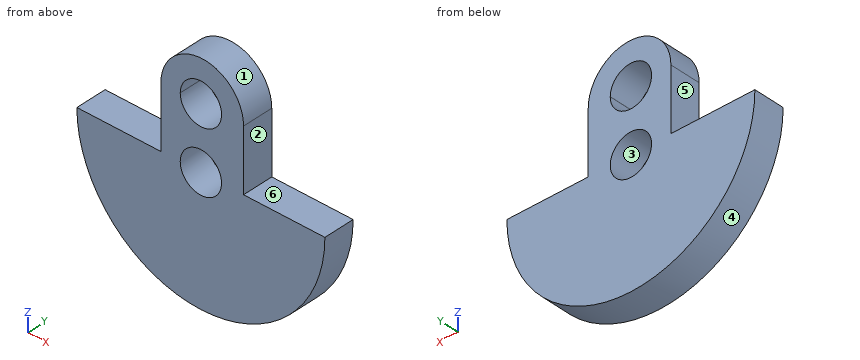
```python
from build123d import *

# Parameters (mm, degrees)
F1_DEPTH = 15


with BuildPart() as f1:
    # F0 (on Front) → F1 (new body)
    with BuildSketch(Plane.XZ):
        with BuildLine():
            Line((-19.364525, 0), (-60, 0))
            ThreePointArc((-60, 0), (0, -60), (60, 0))
            Line((60, 0), (20.64457, 0))
            Line((20.64457, 0), (10, 0))
            ThreePointArc((10, 0), (0, -10), (-10, 0))
            Line((-10, 0), (-19.364525, 0))
        make_face()
        with BuildLine():
            Line((-19.364525, 30.053675), (-19.364525, 0))
            Line((-19.364525, 0), (-10, 0))
            ThreePointArc((-10, 0), (0, 10), (10, 0))
            Line((10, 0), (20.64457, 0))
            Line((20.64457, 0), (20.64457, 30.053675))
            Line((20.64457, 30.053675), (9.999856, 30.053675))
            ThreePointArc((9.999856, 30.053675), (9.999964, 30.026838), (10, 30))
            ThreePointArc((10, 30), (-0.026838, 20.000036), (-9.999856, 30.053675))
            Line((-9.999856, 30.053675), (-19.364525, 30.053675))
        make_face()
        with BuildLine():
            ThreePointArc((20.64457, 30.053675), (0.640023, 50.058223), (-19.364525, 30.053675))
            Line((-19.364525, 30.053675), (-9.999856, 30.053675))
            ThreePointArc((-9.999856, 30.053675), (0, 40), (9.999856, 30.053675))
            Line((9.999856, 30.053675), (20.64457, 30.053675))
        make_face()
    extrude(amount=F1_DEPTH)


solid = f1.part
```
Build history of the part. All positions in model axes, mm. Face numbers are marked on the shaded views. A direction names the side the tool comes from. Round coordinates to 2 decimals unless told otherwise and drop trailing zeros. Write each loop counter-clockwise with the first axis right and the second up, starting at its lowest first coordinate (ties: lowest second). Pieces come first, ordered by that corner, then holes.
1) Band-saw the part on D-D, the plane z = 37.5. List the corners of the cut face in (x, y).
2) Band-saw the part on A-A, the plane y = -4. List the corners of the cut face in (x, z), and give its area (3 significant figures).
3) Pin check, flat tips, straight feed: pin 1 (1 mm diameter, centred on x = 6, y = -2, fed in from +Z); pin 2 (3 mm diameter, centred on x = 3.5, y = -3, fed in from +Z); pin 3 (3 mm diameter, centred on y = -10.5, z = 8, fed in from +X). Stop position of each tip, or through.
4) Drill centre lines: probe 1 along Z at (x, y) = (0, -10.5); probe 2 along Z at (x, y) = (-5, -10.75); probe 3 along X at (y, z) = (-1.5, 17). Where is each one in solid material? Low to high.
5) Mould opens along X. For the marked faces 1, 2 and 3 say: +X half, -X half, draft (parallel to the pull), parting line (faces both ways), or undercut.
6) Band-saw the part on B-B, the plane z = -3. List the corners of the cut face in (x, y).
7) Band-saw the part on C-C, the plane x = -8. List the corners of the cut face in (y, z).
8) 3-axis set-ups, long thin cutter, end or side, ignore diameter. For the marked faces 4, 5 and 6: which of +Z, -Z, +X, -X, +Y, -Y reach the whole face in a straight line?
Ans:
1. outline: (-17.93, -15) - (-6.61, -15) - (-6.61, 0) - (-17.93, 0) - close; (6.61, -15) - (19.21, -15) - (19.21, 0) - (6.61, 0) - close
2. outline: (-60, 0) arc R60 ccw to (60, 0) - (20.64, 0) - (20.64, 30.05) arc R20 ccw to (-19.36, 30.05) - (-19.36, 0) - close; hole circle Ø20 at (0, 0); hole (10, 30) arc R10 ccw to (10, 30.05) arc R10 ccw (long way) to start
2. area: 6,860 mm2
3. pin 1: stops at z = 49.46
3. pin 2: stops at z = 50.01
3. pin 3: stops at x = 20.64
4. probe 1: z = -60 to -10, 10 to 20, 40 to 50.05
4. probe 2: z = -59.79 to -8.66, 8.66 to 21.34, 38.66 to 49.25
4. probe 3: x = -19.36 to 20.64
5. face 1: parting line
5. face 2: +X half
5. face 3: undercut
6. outline: (-59.92, -15) - (-9.54, -15) - (-9.54, 0) - (-59.92, 0) - close; (9.54, -15) - (59.92, -15) - (59.92, 0) - (9.54, 0) - close
7. outline: (-15, -59.46) - (0, -59.46) - (0, -6) - (-15, -6) - close; (-15, 6) - (0, 6) - (0, 24) - (-15, 24) - close; (-15, 36) - (0, 36) - (0, 48.1) - (-15, 48.1) - close
8. face 4: -Z, +Y, -Y
8. face 5: +Z, -X, +Y, -Y
8. face 6: +Z, +X, +Y, -Y
